The model under review builds one solid part; all positions refer to its coordinate system, in mm. A direction names the side the tool comes from. Give positions to 0.01 mm unless a question says otherwise; leave off trailing zeros. Loops run counter-clockwise (first coordinate to the right, second up) from the corner with the lowest first, then second, coordinate; pieces in that order, holes last. Notation, with made-up numbers: (54.5, -9) - (101.5, -9) arc R28 ccw to (101.5, 26) - close; hole circle Ø4 at (28, 75.25). An arc over 180 degrees is marked (long way). Answer as a JSON object with one key per item and string values.
from build123d import *

# Parameters (mm, degrees)
SKETCH_1_W                  = 86
SKETCH_1_H                  = 44.2
EXTRUDE_1_DEPTH             = 14.2
EXTRUDE_2_DEPTH             = 5
SKETCH_3_W                  = 40.1
SKETCH_3_H                  = 42.4
CUT_EXTRUDE_1_DEPTH         = 18.3
SKETCH_4_W                  = 40.1
SKETCH_4_H                  = 42.4
CUT_EXTRUDE_2_DEPTH         = 18.3
HOLE_WIZARD_8_3_8_3_1_D     = 8.3
HOLE_WIZARD_8_3_8_3_1_DEPTH = 3.2
HOLE_WIZARD_6_0_6_1_D       = 6
HOLE_WIZARD_6_0_6_1_DEPTH   = 0.9
FILLET_1_R                  = 3
EXTRUDE_START               = -3.5
SKETCH_9_R                  = 4.15
EXTRUDE_3_DEPTH             = 3.5
FILLET_2_R                  = 2
FILLET_3_R                  = 2
FILLET_4_R                  = 2
FILLET_5_R                  = 2


with BuildPart() as part:
    # Эскиз1 → Бобышка-Вытянуть1 (new body)
    with BuildSketch(Plane.XY.offset(9.6)):
        with Locations((47, 0)):
            Rectangle(SKETCH_1_W, SKETCH_1_H)
    extrude(amount=-EXTRUDE_1_DEPTH)

    # Эскиз2 → Бобышка-Вытянуть2 (add)
    with BuildSketch(Plane(origin=(0, 0, -4.6), x_dir=(-1, 0, 0), z_dir=(0, 0, -1))):
        with BuildLine():
            Line((-90, -22.1), (-90, -17.1))
            ThreePointArc((-90, -17.1), (-104, 0), (-90, 17.1))
            Line((-90, 17.1), (-90, 22.1))
            Line((-90, 22.1), (-4, 22.1))
            Line((-4, 22.1), (-4, -22.1))
            Line((-4, -22.1), (-90, -22.1))
        make_face()
        with BuildLine():
            Line((-90, -12.994779171), (-90, 12.994779171))
            ThreePointArc((-90, 12.994779171), (-100, 0), (-90, -12.994779171))
        make_face(mode=Mode.SUBTRACT)
    extrude(amount=EXTRUDE_2_DEPTH)

    # Эскиз3 → Вырез-Вытянуть1 (cut)
    with BuildSketch(Plane.XY.offset(9.6)):
        with Locations((28.05, 0)):
            Rectangle(SKETCH_3_W, SKETCH_3_H)
    extrude(amount=-CUT_EXTRUDE_1_DEPTH, mode=Mode.SUBTRACT)

    # Эскиз4 → Вырез-Вытянуть2 (cut)
    with BuildSketch(Plane.XY.offset(9.6)):
        with Locations((69.05, 0)):
            Rectangle(SKETCH_4_W, SKETCH_4_H)
    extrude(amount=-CUT_EXTRUDE_2_DEPTH, mode=Mode.SUBTRACT)

    # Диаметр отверстия Ø8.3 (8.3)1
    with Locations(Plane.ZY.offset(-4)):
        with Locations((0, 0)):
            Hole(HOLE_WIZARD_8_3_8_3_1_D / 2, depth=HOLE_WIZARD_8_3_8_3_1_DEPTH)

    # Диаметр отверстия Ø6.0 (6)1
    with Locations(Plane.ZY.offset(-48.1)):
        with Locations((9.6, 0)):
            Hole(HOLE_WIZARD_6_0_6_1_D / 2, depth=HOLE_WIZARD_6_0_6_1_DEPTH)

    # Скругление1
    fillet_1_edges = [part.edges().sort_by_distance(p)[0] for p in [
        (4, -22.1, 0),
        (4, 22.1, 0),
    ]]
    fillet(fillet_1_edges, radius=FILLET_1_R)

    # Эскиз9 → Бобышка-Вытянуть3 (add)
    with BuildSketch(Plane.ZY.offset(-4).offset(EXTRUDE_START)):
        Circle(SKETCH_9_R)
    extrude(amount=EXTRUDE_3_DEPTH)

    # Скругление2
    # the kernel refuses this fillet: 2 mm, written as the material it adds along each edge
    with BuildSketch(Plane(origin=(51, 19.2, -6.7), x_dir=(0, 1, 0), z_dir=(-1, 0, 0))) as fillet_2_piece_1_section:
        Polygon((0, 0), (FILLET_2_R * 1.02, 0), (FILLET_2_R * 1.02, FILLET_2_R * 1.02), (0, FILLET_2_R * 1.02), align=None)
    fillet_2_piece_1 = extrude(amount=FILLET_2_R * 1.02, mode=Mode.PRIVATE)
    fillet_2_piece_1 = fillet_2_piece_1 - Plane(origin=(51, 19.2, -6.7), x_dir=(0, -0.7071067811865475, 0.7071067811865475), z_dir=(-1, 0, 0)) * Sphere(FILLET_2_R, mode=Mode.PRIVATE)
    add(fillet_2_piece_1)
    with BuildSketch(Plane(origin=(46.1, -19.2, -6.7), x_dir=(0, 0, -1), z_dir=(0, -1, 0))) as fillet_2_piece_2_section:
        Polygon((0, 0), (FILLET_2_R * 1.02, 0), (FILLET_2_R * 1.02, FILLET_2_R * 1.02), (0, FILLET_2_R * 1.02), align=None)
    fillet_2_piece_2 = extrude(amount=FILLET_2_R * 1.02, mode=Mode.PRIVATE)
    fillet_2_piece_2 = fillet_2_piece_2 - Plane(origin=(46.1, -19.2, -6.7), x_dir=(-0.7071067811865475, 0, 0.7071067811865475), z_dir=(0, -1, 0)) * Sphere(FILLET_2_R, mode=Mode.PRIVATE)
    add(fillet_2_piece_2)
    with BuildSketch(Plane(origin=(10, -19.2, -6.7), x_dir=(-1, 0, 0), z_dir=(0, 0, -1))) as fillet_2_piece_3_section:
        Polygon((0, 0), (FILLET_2_R * 1.02, 0), (FILLET_2_R * 1.02, -FILLET_2_R * 1.02), (0, -FILLET_2_R * 1.02), align=None)
    fillet_2_piece_3 = extrude(amount=FILLET_2_R * 1.02, mode=Mode.PRIVATE)
    fillet_2_piece_3 = fillet_2_piece_3 - Plane(origin=(10, -19.2, -6.7), x_dir=(0.707106781186543, 0.7071067811865519, 0), z_dir=(0, 0, -1)) * Sphere(FILLET_2_R, mode=Mode.PRIVATE)
    add(fillet_2_piece_3)
    with BuildSketch(Plane(origin=(10, 19.2, -6.7), x_dir=(0, 1, 0), z_dir=(0, 0, -1))) as fillet_2_piece_4_section:
        Polygon((0, 0), (FILLET_2_R * 1.02, 0), (FILLET_2_R * 1.02, -FILLET_2_R * 1.02), (0, -FILLET_2_R * 1.02), align=None)
    fillet_2_piece_4 = extrude(amount=FILLET_2_R * 1.02, mode=Mode.PRIVATE)
    fillet_2_piece_4 = fillet_2_piece_4 - Plane(origin=(10, 19.2, -6.7), x_dir=(0.7071067811865475, -0.7071067811865475, 0), z_dir=(0, 0, -1)) * Sphere(FILLET_2_R, mode=Mode.PRIVATE)
    add(fillet_2_piece_4)
    with BuildSketch(Plane(origin=(89.1, -21.2, -8.7), x_dir=(0, 0, 1), z_dir=(0, 1, 0))) as fillet_2_piece_5:
        with BuildLine():
            CenterArc((FILLET_2_R, -FILLET_2_R), FILLET_2_R, 90, 90)
            Line((0, -FILLET_2_R), (0, 0))
            Line((0, 0), (FILLET_2_R, 0))
        make_face()
    extrude(amount=42.4)
    with BuildSketch(Plane(origin=(89.1, 21.2, -8.7), x_dir=(0, 0, 1), z_dir=(-1, 0, 0))) as fillet_2_piece_6:
        with BuildLine():
            CenterArc((FILLET_2_R, -FILLET_2_R), FILLET_2_R, 90, 90)
            Line((0, -FILLET_2_R), (0, 0))
            Line((0, 0), (FILLET_2_R, 0))
        make_face()
    extrude(amount=38.1)
    with BuildSketch(Plane(origin=(49, 21.2, 9.6), x_dir=(0, -1, 0), z_dir=(0, 0, -1)), Plane(origin=(48.1, -21.2, 9.6), x_dir=(0, 1, 0), z_dir=(0, 0, -1))) as fillet_2_piece_7:
        with BuildLine():
            CenterArc((FILLET_2_R, -FILLET_2_R), FILLET_2_R, 90, 90)
            Line((0, -FILLET_2_R), (0, 0))
            Line((0, 0), (FILLET_2_R, 0))
        make_face()
    extrude(amount=16.3)
    with BuildSketch(Plane(origin=(8, -21.2, 9.6), x_dir=(0, 1, 0), z_dir=(0, 0, -1)), Plane(origin=(8, 21.2, 9.6), x_dir=(1, 0, 0), z_dir=(0, 0, -1))) as fillet_2_piece_8:
        with BuildLine():
            CenterArc((FILLET_2_R, FILLET_2_R), FILLET_2_R, 180, 90)
            Line((0, FILLET_2_R), (0, 0))
            Line((0, 0), (FILLET_2_R, 0))
        make_face()
    extrude(amount=16.3)
    with BuildSketch(Plane(origin=(49, 19.2, -8.7), x_dir=(0, 0, 1), z_dir=(0, -1, 0)), Plane(origin=(48.1, -19.2, -8.7), x_dir=(0, 0, 1), z_dir=(0, 1, 0))) as fillet_2_piece_9:
        with BuildLine():
            CenterArc((FILLET_2_R, -FILLET_2_R), FILLET_2_R, 90, 90)
            Line((0, -FILLET_2_R), (0, 0))
            Line((0, 0), (FILLET_2_R, 0))
        make_face()
    extrude(amount=40.4)
    with BuildSketch(Plane(origin=(53.1, 21.2, -8.7), x_dir=(0, 0, 1), z_dir=(-1, 0, 0))) as fillet_2_piece_10:
        with BuildLine():
            CenterArc((FILLET_2_R, -FILLET_2_R), FILLET_2_R, 90, 90)
            Line((0, -FILLET_2_R), (0, 0))
            Line((0, 0), (FILLET_2_R, 0))
        make_face()
    extrude(amount=43.1)
    with BuildSketch(Plane(origin=(10, -21.2, -8.7), x_dir=(0, 0, 1), z_dir=(1, 0, 0))) as fillet_2_piece_11:
        with BuildLine():
            CenterArc((FILLET_2_R, -FILLET_2_R), FILLET_2_R, 90, 90)
            Line((0, -FILLET_2_R), (0, 0))
            Line((0, 0), (FILLET_2_R, 0))
        make_face()
    extrude(amount=36.1)
    with BuildSketch(Plane(origin=(8, 19.2, -8.7), x_dir=(0, 0, 1), z_dir=(0, -1, 0))) as fillet_2_piece_12:
        with BuildLine():
            CenterArc((FILLET_2_R, -FILLET_2_R), FILLET_2_R, 90, 90)
            Line((0, -FILLET_2_R), (0, 0))
            Line((0, 0), (FILLET_2_R, 0))
        make_face()
    extrude(amount=38.4)
    # the kernel refuses this fillet: 2 mm, written as the material it takes off along each edge
    with BuildSketch(Plane(origin=(49, -21.2, 9.6), x_dir=(0, -1, 0), z_dir=(1, 0, 0))) as fillet_2_2_piece_1:
        with BuildLine():
            CenterArc((FILLET_2_R, FILLET_2_R), FILLET_2_R, 180, 90)
            Line((0, FILLET_2_R), (0, 0))
            Line((0, 0), (FILLET_2_R, 0))
        make_face()
    extrude(amount=40.1, mode=Mode.SUBTRACT)

    # Скругление3
    # the kernel refuses this fillet: 2 mm, written as the material it adds along each edge
    with BuildSketch(Plane(origin=(46.1, 19.2, -6.7), x_dir=(0, 1, 0), z_dir=(1, 0, 0))) as fillet_3_piece_1_section:
        Polygon((0, 0), (FILLET_3_R, 0), (FILLET_3_R, -FILLET_3_R), (0, -FILLET_3_R), align=None)
    fillet_3_piece_1 = extrude(amount=FILLET_3_R, mode=Mode.PRIVATE)
    fillet_3_piece_1 = fillet_3_piece_1 - Plane(origin=(46.1, 19.2, -6.7), x_dir=(0, -0.7071067811865475, 0.7071067811865475), z_dir=(1, 0, 0)) * Sphere(FILLET_3_R, mode=Mode.PRIVATE)
    add(fillet_3_piece_1)
    with BuildSketch(Plane(origin=(89.1, -23.2, 7.6), x_dir=(0, 1, 0), z_dir=(0, 0, -1))) as fillet_3_piece_2_section:
        with BuildLine():
            CenterArc((2 + FILLET_3_R, -FILLET_3_R), FILLET_3_R, 90, 90)
            Line((2, -FILLET_3_R), (2, 0))
            Line((2, 0), (2 + FILLET_3_R, 0))
        make_face()
    fillet_3_piece_2 = revolve(axis=Axis((89.1, -23.2, 7.6), (1, 0, 0)), revolution_arc=199.895215799, mode=Mode.PRIVATE)
    fillet_3_piece_2 = split(fillet_3_piece_2, bisect_by=Plane(origin=(88.655987969, -22.1, 8.63173809), z_dir=(0, 1, 0)), keep=Keep.TOP, mode=Mode.PRIVATE)
    fillet_3_piece_2 = split(fillet_3_piece_2, bisect_by=Plane(origin=(88.655987969, -21.07116748, 9.6), z_dir=(0, 0, -1)), keep=Keep.TOP, mode=Mode.PRIVATE)
    add(fillet_3_piece_2)
    with BuildSketch(Plane(origin=(89.1, -21.2, 7.6), x_dir=(0, 1, 0), z_dir=(0, 0, -1))) as fillet_3_piece_3:
        with BuildLine():
            CenterArc((FILLET_3_R, -FILLET_3_R), FILLET_3_R, 90, 90)
            Line((0, -FILLET_3_R), (0, 0))
            Line((0, 0), (FILLET_3_R, 0))
        make_face()
    extrude(amount=14.3)
    with BuildSketch(Plane(origin=(87.1, -21.2, -6.7), x_dir=(1, 0, 0), z_dir=(0, 0, 1))) as fillet_3_piece_4:
        with BuildLine():
            CenterArc((2 - FILLET_3_R, FILLET_3_R), FILLET_3_R, 270, 90)
            Line((2 - FILLET_3_R, 0), (2, 0))
            Line((2, 0), (2, FILLET_3_R))
        make_face()
    revolve(axis=Axis((87.1, -21.2, -6.7), (0, 1, 0)), revolution_arc=90)
    with BuildSketch(Plane(origin=(51, -21.2, -8.7), x_dir=(0, 1, 0), z_dir=(1, 0, 0))) as fillet_3_piece_5:
        with BuildLine():
            CenterArc((FILLET_3_R, FILLET_3_R), FILLET_3_R, 180, 90)
            Line((0, FILLET_3_R), (0, 0))
            Line((0, 0), (FILLET_3_R, 0))
        make_face()
    extrude(amount=36.1)
    with BuildSketch(Plane(origin=(51, -21.2, -6.7), x_dir=(-1, 0, 0), z_dir=(0, 0, 1))) as fillet_3_piece_6:
        with BuildLine():
            CenterArc((2 - FILLET_3_R, -FILLET_3_R), FILLET_3_R, 360, 90)
            Line((2, -FILLET_3_R), (2, 0))
            Line((2, 0), (2 - FILLET_3_R, 0))
        make_face()
    revolve(axis=Axis((51, -21.2, -6.7), (0, -1, 0)), revolution_arc=90)
    with BuildSketch(Plane(origin=(49, -23.2, 7.6), x_dir=(0, 1, 0), z_dir=(0, 0, -1))) as fillet_3_piece_7_section:
        with BuildLine():
            CenterArc((2 + FILLET_3_R, FILLET_3_R), FILLET_3_R, 180, 90)
            Line((2, FILLET_3_R), (2, 0))
            Line((2, 0), (2 + FILLET_3_R, 0))
        make_face()
    fillet_3_piece_7 = revolve(axis=Axis((49, -23.2, 7.6), (1, 0, 0)), revolution_arc=199.895215799, mode=Mode.PRIVATE)
    fillet_3_piece_7 = split(fillet_3_piece_7, bisect_by=Plane(origin=(49.444012031, -22.1, 8.63173809), z_dir=(0, 1, 0)), keep=Keep.TOP, mode=Mode.PRIVATE)
    fillet_3_piece_7 = split(fillet_3_piece_7, bisect_by=Plane(origin=(49.444012031, -21.07116748, 9.6), z_dir=(0, 0, -1)), keep=Keep.TOP, mode=Mode.PRIVATE)
    add(fillet_3_piece_7)
    with BuildSketch(Plane(origin=(49, -21.2, 7.6), x_dir=(0, 1, 0), z_dir=(0, 0, -1))) as fillet_3_piece_8:
        with BuildLine():
            CenterArc((FILLET_3_R, FILLET_3_R), FILLET_3_R, 180, 90)
            Line((0, FILLET_3_R), (0, 0))
            Line((0, 0), (FILLET_3_R, 0))
        make_face()
    extrude(amount=14.3)
    with BuildSketch(Plane(origin=(48.1, 21.2, 9.6), x_dir=(0, -1, 0), z_dir=(0, 0, -1))) as fillet_3_piece_9:
        with BuildLine():
            CenterArc((FILLET_3_R, FILLET_3_R), FILLET_3_R, 180, 90)
            Line((0, FILLET_3_R), (0, 0))
            Line((0, 0), (FILLET_3_R, 0))
        make_face()
    extrude(amount=16.3)

    # Скругление4
    # the kernel refuses this fillet: 2 mm, written as the material it adds along each edge
    with BuildSketch(Plane(origin=(87.1, 19.2, -6.7), x_dir=(0, 1, 0), z_dir=(1, 0, 0))) as fillet_4_piece_1_section:
        Polygon((0, 0), (FILLET_4_R, 0), (FILLET_4_R, -FILLET_4_R), (0, -FILLET_4_R), align=None)
    fillet_4_piece_1 = extrude(amount=FILLET_4_R, mode=Mode.PRIVATE)
    fillet_4_piece_1 = fillet_4_piece_1 - Plane(origin=(87.1, 19.2, -6.7), x_dir=(0, -0.7071067811865475, 0.7071067811865475), z_dir=(1, 0, 0)) * Sphere(FILLET_4_R, mode=Mode.PRIVATE)
    add(fillet_4_piece_1)
    with BuildSketch(Plane(origin=(89.1, 21.2, 9.6), x_dir=(0, -1, 0), z_dir=(0, 0, -1))) as fillet_4_piece_2:
        with BuildLine():
            CenterArc((FILLET_4_R, FILLET_4_R), FILLET_4_R, 180, 90)
            Line((0, FILLET_4_R), (0, 0))
            Line((0, 0), (FILLET_4_R, 0))
        make_face()
    extrude(amount=16.3)

    # Скругление5
    fillet_5_edges = [part.edges().sort_by_distance(p)[0] for p in [
        (90, -15.047389586, -4.6),
        (90, 15.047389586, -4.6),
    ]]
    fillet(fillet_5_edges, radius=FILLET_5_R)


solid = part.part
Q1. Clearance check with flat-ended pins moving along their axes: pin 1 Ø10 at (y, z) = (-5, 0) entering from +X; pin 2 Ø1 at (y, z) = (17, 2.5) entering from +X; pin 3 Ø5 at (y, z) = (-6.5, -2.5) entering from +X. State where each tip first meets the part, or that it passes through.
Results:
{"pin 1": "stops at x = 103.73", "pin 2": "stops at x = 90", "pin 3": "stops at x = 103.22"}
Q2. Consider section D-D, the plane y = 8. State the section outline as (x, z) points.
Results:
{"outline": "(4, -9.6) - (90, -9.6) - (90, 9.6) - (89.1, 9.6) - (89.1, -6.7) arc R2 cw to (87.1, -8.7) - (51, -8.7) arc R2 cw to (49, -6.7) - (49, 9.6) - (48.1, 9.6) - (48.1, -6.7) arc R2 cw to (46.1, -8.7) - (10, -8.7) arc R2 cw to (8, -6.7) - (8, 9.6) - (4, 9.6) - close; (97.36, -9.6) - (102.06, -9.6) - (102.06, -4.6) - (97.36, -4.6) - close"}
Q3. Consider section A-A, the plane y = 0. State the section outline as (x, z) points.
Results:
{"outline": "(4, -9.6) - (90, -9.6) - (90, 9.6) - (89.1, 9.6) - (89.1, -6.7) arc R2 cw to (87.1, -8.7) - (51, -8.7) arc R2 cw to (49, -6.7) - (49, 6.6) - (48.1, 6.6) - (48.1, -6.7) arc R2 cw to (46.1, -8.7) - (10, -8.7) arc R2 cw to (8, -6.7) - (8, 9.6) - (4, 9.6) - close; (100, -9.6) - (104, -9.6) - (104, -4.6) - (100, -4.6) - close"}
Q4. Consider section C-C, the plane z = 4.25. State the section outline as (x, y) points, plus the area to 3 significant figures.
Results:
{"outline": "(4, -19.1) arc R3 ccw to (7, -22.1) - (90, -22.1) - (90, 22.1) - (7, 22.1) arc R3 ccw to (4, 19.1) - close; hole (8, -19.2) arc R2 ccw to (10, -21.2) - (46.1, -21.2) arc R2 ccw to (48.1, -19.2) - (48.1, 19.2) arc R2 ccw to (46.1, 21.2) - (10, 21.2) arc R2 ccw to (8, 19.2) - close; hole (49, -19.2) arc R2 ccw to (51, -21.2) - (87.1, -21.2) arc R2 ccw to (89.1, -19.2) - (89.1, 19.2) arc R2 ccw to (87.1, 21.2) - (51, 21.2) arc R2 ccw to (49, 19.2) - close", "area": "404 mm^2"}
Q5. To check wall thickness, follow probe 1 along X at (y, z) = (-12, 3); probe 2 along Y at (x, z) = (84, 0.25); probe 3 along X at (y, z) = (-14, -6). State the ranges of each line that lie inside material, in increasing order. Write a range as [from, to].
Results:
{"probe 1": "x = [4, 8], [48.1, 49], [89.1, 90]", "probe 2": "y = [-22.1, -21.2], [21.2, 22.1]", "probe 3": "x = [4, 8], [48.1, 49], [89.1, 96.96]"}
Q6. For faces 5 (the face through (48, 22.1, 0)), 6 (the face through (68.797, -21.433, 8.536)), list the 3-axis set-ups (+Z, -Z, +X, -X, +Y, -Y) from which the entire face can be reached by the end or side of a thin tool; tool diameter is ignored.
Results:
{"face 5": "+Z, -Z, +X, -X, +Y", "face 6": "+Z"}
Q7. The part is to be moulded in two halves that separate along Y. For faces 1 (the face through (27.8, -20.63, -8.1)), 2 (the face through (4.9, -21.24, -0.13)), 3 (the face through (8.6, -20.63, 1.56)), 4 (the face through (5, -5, 9.6)), say which applies: +Y half, -Y half, draft (parallel to the pull), parting line (faces both ways), or undercut.
Results:
{"face 1": "undercut", "face 2": "-Y half", "face 3": "undercut", "face 4": "draft"}
Q8. Consider section B-B, the plane x = 22. State the section outline as (y, z) points.
Results:
{"outline": "(-22.1, -9.6) - (22.1, -9.6) - (22.1, 9.6) - (21.2, 9.6) - (21.2, -6.7) arc R2 cw to (19.2, -8.7) - (-19.2, -8.7) arc R2 cw to (-21.2, -6.7) - (-21.2, 9.6) - (-22.1, 9.6) - close"}
